Geometry: final body of the model. Coordinates: model frame, mm. Face numbers are marked on the shaded views. Coordinates: 2 decimals unless noted, no trailing zeros. Write each loop counter-clockwise with the first axis right and the second up, starting at its lowest first coordinate (ties: lowest second). Pieces come first, ordered by that corner, then holes. Notation, with made-up numbers: M -13,85.25 L 36,85.25 A15 cw 36,97.25 Z; hole C 58,-11 d4. An arc over 180 degrees is marked long. Write item = value, one per line. Start each with the question number.
Item 1: Section A-A on x = 115. Output: boundary loops of the cut face in (y, z), plus the area to 3 significant figures.
Item 2: Section C-C on z = 2.1. Give the number of separate pieces and of enclosed holes in the cut face, plus the area to 3 significant figures.
Item 3: Section B-B on y = -13. Output: boundary loops of the cut face in (x, z), plus the area to 3 significant figures.
Item 4: Ray query, L1, parallel to Y at x = -56, z = 1.7; L2, parallel to Y at x = 218, z = 3.1; L3, parallel to Y at x = -109, z = 2.3. Return the intervals inside material, ascending. Write a range as [from, to].
Item 5: Pull-direction query (Z, two-part tool) for the marked faces 1 and 2; classes: +Z half, -Z half, draft (parallel to the pull), parting line (faces both ways), or undercut.
Item 6: First-contact query: pin 1 Ø2.5 at (x, y) = (-134, -103) entering from -Z. Flat tip, straight axial feed; report the tip coordinate or a pass-through.
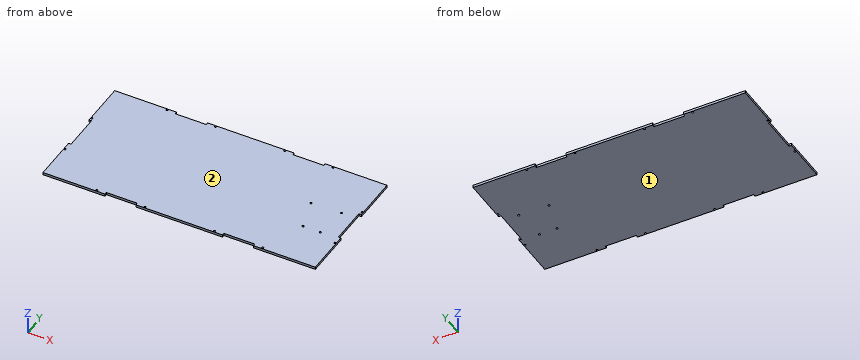
from build123d import *

# Parameters (mm, degrees)
ESQUISSE1_W             = 440
ESQUISSE1_H             = 210
BOSS_EXTRU_1_DEPTH      = 4
ESQUISSE2_W             = 50
ESQUISSE2_H             = 4
ESQUISSE2_W_2           = 4
ESQUISSE2_H_2           = 60
ENL_V_MAT_EXTRU_1_DEPTH = 4
ESQUISSE4_R             = 1.6
ENL_V_MAT_EXTRU_2_DEPTH = 10
ESQUISSE5_R             = 1.5875
ESQUISSE5_R_2           = 1.598396888
ENL_V_MAT_EXTRU_3_DEPTH = 4


with BuildPart() as part:
    # Esquisse1 → Boss.-Extru.1 (new body)
    with BuildSketch(Plane.XY):
        Rectangle(ESQUISSE1_W, ESQUISSE1_H)
    extrude(amount=BOSS_EXTRU_1_DEPTH)

    # Esquisse2 → Enlèv. mat.-Extru.1 (cut)
    with BuildSketch(Plane.XY.offset(4)):
        with Locations((-95, 103)):
            Rectangle(ESQUISSE2_W, ESQUISSE2_H)
        with Locations((95, 103)):
            Rectangle(ESQUISSE2_W, ESQUISSE2_H)
        with Locations((218, 0)):
            Rectangle(ESQUISSE2_W_2, ESQUISSE2_H_2)
        with Locations((-218, 0)):
            Rectangle(ESQUISSE2_W_2, ESQUISSE2_H_2)
        with Locations((95, -103)):
            Rectangle(ESQUISSE2_W, ESQUISSE2_H)
        with Locations((-95, -103)):
            Rectangle(ESQUISSE2_W, ESQUISSE2_H)
    extrude(amount=-ENL_V_MAT_EXTRU_1_DEPTH, mode=Mode.SUBTRACT)

    # Esquisse4 → Enlèv. mat.-Extru.2 (cut)
    with BuildSketch(Plane.XY.offset(4)):
        with Locations((218, -44)):
            Circle(ESQUISSE4_R)
        with Locations((218.375135888, 35)):
            Circle(ESQUISSE4_R)
        with Locations((-56, 103)):
            Circle(ESQUISSE4_R)
        with Locations((-134, 103)):
            Circle(ESQUISSE4_R)
        with Locations((-218.375135888, 35)):
            Circle(ESQUISSE4_R)
        with Locations((-56, -103)):
            Circle(ESQUISSE4_R)
        with Locations((-134, -103)):
            Circle(ESQUISSE4_R)
        with Locations((134, 103)):
            Circle(ESQUISSE4_R)
        with Locations((56, 103)):
            Circle(ESQUISSE4_R)
        with Locations((-218, -44)):
            Circle(ESQUISSE4_R)
        with Locations((56, -103)):
            Circle(ESQUISSE4_R)
        with Locations((134, -103)):
            Circle(ESQUISSE4_R)
    extrude(amount=-ENL_V_MAT_EXTRU_2_DEPTH, mode=Mode.SUBTRACT)

    # Esquisse5 → Enlèv. mat.-Extru.3 (cut)
    with BuildSketch(Plane(origin=(0, 0, 0), x_dir=(-1, 0, 0), z_dir=(0, 0, -1))):
        with Locations((-145.216701852, 18.010439522)):
            Circle(ESQUISSE5_R)
        with Locations((-160.435580246, -32.780039682)):
            Circle(ESQUISSE5_R_2)
        with Locations((-188.38, -32.79)):
            Circle(ESQUISSE5_R)
        with Locations((-193.46, 19.28)):
            Circle(ESQUISSE5_R)
    extrude(amount=-ENL_V_MAT_EXTRU_3_DEPTH, mode=Mode.SUBTRACT)


solid = part.part
Responses:
q1.outline = M -101,0 L 101,0 L 101,4 L -101,4 Z
q1.area = 808 mm²
q2.separate_pieces = 1
q2.enclosed_holes = 16
q2.area = 91,000 mm²
q3.outline = M -216,0 L 216,0 L 216,4 L -216,4 Z
q3.area = 1,730 mm²
q4.L1 = [-105, -104.6], [-101.4, 101.4], [104.6, 105]
q4.L2 = [-105, -45.6], [-42.4, -30], [30, 33.44], [36.56, 105]
q4.L3 = [-101, 101]
q5.face_1 = -Z half
q5.face_2 = +Z half
q6.pin_1 = through
